```python
from build123d import *

# Parameters (mm, degrees)
VISTA_FRONTAL_W       = 59.6
VISTA_FRONTAL_H       = 28
VISTA_FRONTAL_W_2     = 54.6
VISTA_FRONTAL_H_2     = 23
CORPO_DO_MODULO_DEPTH = 15.8
ESBO_O3_R             = 1.3
CORTE_EXTRUS_O1_DEPTH = 44.836970698
ESBO_O4_R             = 2
ESBO_O4_W             = 3
ESBO_O4_H             = 17
CORTE_EXTRUS_O2_DEPTH = 3.6


with BuildPart() as part:
    # Vista Frontal → Corpo do Modulo (new, symmetric)
    with BuildSketch(Plane.XY):
        Rectangle(VISTA_FRONTAL_W, VISTA_FRONTAL_H)
        Rectangle(VISTA_FRONTAL_W_2, VISTA_FRONTAL_H_2, mode=Mode.SUBTRACT)
    extrude(amount=CORPO_DO_MODULO_DEPTH, both=True)

    # Esboço3 → Corte-extrusão1 (cut, through all)
    with BuildSketch(Plane(origin=(0, 14, 0), x_dir=(1, 0, 0), z_dir=(0, 1, 0))):
        with Locations((-29.8, 0)):
            Circle(ESBO_O3_R)
        Polygon((26.970983681, -15.8), (29.8, -10.9), (29.8, -15.8), align=None)
        Polygon((29.8, 15.8), (26.970983681, 15.8), (29.8, 10.9), align=None)
    extrude(amount=-CORTE_EXTRUS_O1_DEPTH, mode=Mode.SUBTRACT)

    # Esboço4 → Corte-extrusão2 (cut)
    with BuildSketch(Plane.XZ.offset(14)):
        with Locations(Location((0, 0, 0), (0, 0, 270))):
            Circle(ESBO_O4_R)
        with Locations(Location((-3, 9.5, 0), (0, 0, 270))):
            Circle(ESBO_O4_R)
        with Locations(Location((-13, 9.5, 0), (0, 0, 270))):
            Circle(ESBO_O4_R)
        with Locations(Location((-13, 3.5, 0), (0, 0, 270))):
            Circle(ESBO_O4_R)
        with Locations(Location((-13, -3.5, 0), (0, 0, 90))):
            Circle(ESBO_O4_R)
        with Locations(Location((-13, -9.5, 0), (0, 0, 90))):
            Circle(ESBO_O4_R)
        with Locations(Location((-3, -9.5, 0), (0, 0, 90))):
            Circle(ESBO_O4_R)
        with Locations((4.5, 0)):
            Rectangle(ESBO_O4_W, ESBO_O4_H)
    extrude(amount=-CORTE_EXTRUS_O2_DEPTH, mode=Mode.SUBTRACT)


solid = part.part
```
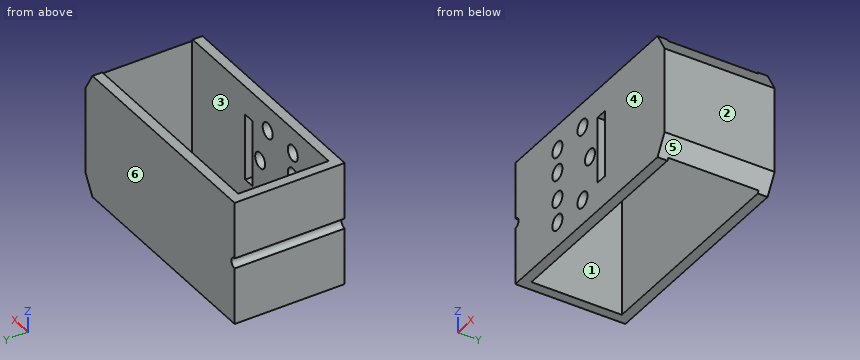
Build history of the part. All positions in model axes, mm. Face numbers are marked on the shaded views. A direction names the side the tool comes from. Round coordinates to 2 decimals unless told otherwise and drop trailing zeros. Write each loop counter-clockwise with the first axis right and the second up, starting at its lowest first coordinate (ties: lowest second). Pieces come first, ordered by that corner, then holes. Notation, with made-up numbers: (85, 33) -> (105, 33) arc R31 ccw to (105, 63) -> close; hole circle Ø11 at (49, 78). An arc over 180 degrees is marked (long way). Put each result on its own line as item: value.
Item 1: Two-plate mould, pull along Y, no slides. Class the marked faces 3, 4, 5 and 6: pulls with the +Y half, pulls with the -Y half, needs draft (parallel to the pull), parting line crosses it, or undercut.
Here are the results:
face 3: undercut
face 4: pulls with the -Y half
face 5: needs draft
face 6: pulls with the +Y half
Item 2: Slice it at A-A, the plane x = 26. Give the cut face in (y, z), plus the area to 3 significant figures.
Here are the results:
outline: (-14, -15.8) -> (-11.5, -15.8) -> (-11.5, 15.8) -> (-14, 15.8) -> close; (11.5, -15.8) -> (14, -15.8) -> (14, 15.8) -> (11.5, 15.8) -> close
area: 158 mm^2
Item 3: Slice it at D-D, the plane z = 3.5. Give the cut face in (x, y), plus the area to 4 significant figures.
Here are the results:
outline: (-29.8, -14) -> (-15, -14) -> (-15, -11.5) -> (-27.3, -11.5) -> (-27.3, 11.5) -> (27.3, 11.5) -> (27.3, -11.5) -> (6, -11.5) -> (6, -14) -> (29.8, -14) -> (29.8, 14) -> (-29.8, 14) -> close; (-11, -14) -> (3, -14) -> (3, -11.5) -> (-11, -11.5) -> close
area: 395.5 mm^2
Item 4: Slice it at C-C, the plane x = -3. Give the cut face in (y, z).
Here are the results:
outline: (-14, -15.8) -> (-11.5, -15.8) -> (-11.5, -11.5) -> (-14, -11.5) -> close; (-14, -7.5) -> (-11.5, -7.5) -> (-11.5, 7.5) -> (-14, 7.5) -> close; (-14, 11.5) -> (-11.5, 11.5) -> (-11.5, 15.8) -> (-14, 15.8) -> close; (11.5, -15.8) -> (14, -15.8) -> (14, 15.8) -> (11.5, 15.8) -> close
Item 5: Slice it at B-B, the plane y = -2. Give the cut face in (x, z), plus the area to 3 significant figures.
Here are the results:
outline: (-29.8, -15.8) -> (-27.3, -15.8) -> (-27.3, 15.8) -> (-29.8, 15.8) -> (-29.8, 1.3) arc R1.3 cw to (-29.8, -1.3) -> close; (27.3, -15.23) -> (29.8, -10.9) -> (29.8, 10.9) -> (27.3, 15.23) -> close
area: 142 mm^2
Item 6: Flat gauge pins, fed straight in: P1, Ø4, axis at x = 2.5, y = 10.5, coming from the -Z side; P2, Ø3, axis at x = 0, z = 0, coming from the -Y side. Where does each tip first touch, or does it go through?
Here are the results:
P1: stops at z = -15.8
P2: stops at y = 11.5
Item 7: Wall check: probe 1 along X at (y, z) = (-12.3, 0); probe 2 along X at (y, z) = (-12.05, -9.5); probe 3 along Y at (x, z) = (-4, -6.5). Give the ranges that are in metal, low to high. Write a range as from..to.
Here are the results:
probe 1: x = -28.5..-2, 2..3, 6..29.8
probe 2: x = -29.8..-15, -11..-5, -1..29.8
probe 3: y = -14..-11.5, 11.5..14
Item 8: Tool access for the marked faces 1 and 2: list every direction of +Z, -Z, +X, -X, +Y, -Y with a clear straight run to the whole face (end or side of a thin tool).
Here are the results:
face 1: +Z, -Z
face 2: +Z, -Z, +X, +Y, -Y
